from build123d import *

# Parameters (mm, degrees)
ESQUISSE2_R        = 18
ESQUISSE2_R_2      = 10.5
BOSS_EXTRU_1_DEPTH = 12


with BuildPart() as part:
    # Esquisse2 → Boss.-Extru.1 (new body)
    with BuildSketch(Plane(origin=(0, 0, 0), x_dir=(1, 0, 0), z_dir=(0, 1, 0))):
        Circle(ESQUISSE2_R)
        with Locations(Location((0, 0, 0), (0, 0, 270))):  # turned: the seam where the file's is
            Circle(ESQUISSE2_R_2, mode=Mode.SUBTRACT)
        with BuildLine():
            Line((-4.75, -17.361955535), (-4.75, -22))
            Line((-4.75, -22), (4.75, -22))
            Line((4.75, -22), (4.75, -17.361955535))
            ThreePointArc((4.75, -17.361955535), (0, -18), (-4.75, -17.361955535))
        make_face()
        with BuildLine():
            Line((-4.75, 27), (-4.75, 17.361955535))
            ThreePointArc((-4.75, 17.361955535), (0, 18), (4.75, 17.361955535))
            Line((4.75, 17.361955535), (4.75, 27))
            Line((4.75, 27), (-4.75, 27))
        make_face()
    extrude(amount=BOSS_EXTRU_1_DEPTH)


solid = part.part
Read the model definition and answer for the solid it produces. Units are mm, in the model's axes. A direction names the side the tool comes from. Round coordinates to 2 decimals unless told otherwise and drop trailing zeros. Write each loop counter-clockwise with the first axis right and the second up, starting at its lowest first coordinate (ties: lowest second). Pieces come first, ordered by that corner, then holes. Notation, with made-up numbers: M 40,52.25 L 51,52.25 A15 ccw 51,72.25 Z; hole C 17.5,58.25 d3. An arc over 180 degrees is marked long. Use a Markdown table: item, result.
1) The part is cut by section A-A (z = 0). Write down the section's boundary in (x, y), plus the area to 3 significant figures.
Answers follow:
| item | result |
|---|---|
| outline | M -18,0 L -10.5,0 L -10.5,12 L -18,12 Z; M 10.5,0 L 18,0 L 18,12 L 10.5,12 Z |
| area | 180 mm2 |
2) Flat-ended cylindrical pins translate along their axes: pin 1 (1.4 mm diameter, centred on y = 6, z = 20, fed in from -X); pin 2 (3 mm diameter, centred on y = 8, z = 16, fed in from -X); pin 3 (5 mm diameter, centred on y = 5.5, z = 19, fed in from +X); pin 4 (5 mm diameter, centred on x = -13.5, z = 16, fed in from +Y). Find the tip coordinate at first contact, or state that the pin passes through.
Answers follow:
| item | result |
|---|---|
| pin 1 | stops at x = -4.75 |
| pin 2 | stops at x = -10.67 |
| pin 3 | stops at x = 7.19 |
| pin 4 | passes through |
3) The part is cut by section B-B (y = 1.25). Write down the section's boundary in (x, z), plus the area to 3 significant figures.
Answers follow:
| item | result |
|---|---|
| outline | M -4.75,-27 L 4.75,-27 L 4.75,-17.36 A18 ccw 4.75,17.36 L 4.75,22 L -4.75,22 L -4.75,17.36 A18 ccw -4.75,-17.36 Z; hole C 0,0 d21 |
| area | 799 mm2 |
4) Straight lines are drawn through the part: line 1 along X through (y, z) = (1, -0.5); line 2 along X through (y, z) = (2, 20); line 3 along Z through (x, y) = (-7, 5). For each, find the intervals that lie inside material, in ascending order. Write a range as [from, to].
Answers follow:
| item | result |
|---|---|
| line 1 | x = [-17.99, -10.49], [10.49, 17.99] |
| line 2 | x = [-4.75, 4.75] |
| line 3 | z = [-16.58, -7.83], [7.83, 16.58] |
5) For a pull along Y with two mould halves and no side action, classify faces 1 (the flat face through (8, 12, -8)), 2 (the flat face through (-4.75, 6, 20)), 3 (the flat face through (8, 0, -8)) as pulls with the +Y half, pulls with the -Y half, needs draft (parallel to the pull), parting line crosses it, or undercut.
Answers follow:
| item | result |
|---|---|
| face 1 | pulls with the +Y half |
| face 2 | needs draft |
| face 3 | pulls with the -Y half |
6) The part is cut by section C-C (x = 0). Write down the section's boundary in (y, z).
Answers follow:
| item | result |
|---|---|
| outline | M 0,-27 L 12,-27 L 12,-10.5 L 0,-10.5 Z; M 0,10.5 L 12,10.5 L 12,22 L 0,22 Z |
7) A tool of negligible diameter and unlimited length cuts with its end or side. For faces 4 (the flat face through (-4.75, 6, -22)), 5 (the flat face through (4.75, 6, 20)), 6 (the flat face through (4.75, 6, -22)), from which of +Z, -Z, +X, -X, +Y, -Y can it reach the whole face along a straight path? Write none if from no direction.
Answers follow:
| item | result |
|---|---|
| face 4 | -Z, -X, +Y, -Y |
| face 5 | +Z, +X, +Y, -Y |
| face 6 | -Z, +X, +Y, -Y |
8) The part is cut by section D-D (z = -23). Write down the section's boundary in (x, y), plus the area to 3 significant figures.
Answers follow:
| item | result |
|---|---|
| outline | M -4.75,0 L 4.75,0 L 4.75,12 L -4.75,12 Z |
| area | 114 mm2 |
